```python
from build123d import *

# Parameters (mm, degrees)
F1_DEPTH = 25.4
F2_DEPTH = 31.75
F3_R     = 8.4375422203
F3_R_2   = 8.3190886378
F4_DEPTH = 74.422


with BuildPart() as f1:
    # F0 (on Front) → F1 (new body, symmetric)
    with BuildSketch(Plane.XZ):
        with BuildLine():
            Line((-29.9681008023, 26.6969427466), (-56.9970235229, 26.6969427466))
            Line((-56.9970235229, 26.6969427466), (-56.9970235229, -26.6969427466))
            Line((-56.9970235229, -26.6969427466), (56.9970235229, -26.6969427466))
            Line((56.9970235229, -26.6969427466), (56.9970235229, 26.6969427466))
            Line((56.9970235229, 26.6969427466), (29.9681008023, 26.6969427466))
            ThreePointArc((29.9681008023, 26.6969427466), (0, -3.2711580556), (-29.9681008023, 26.6969427466))
        make_face()
    extrude(amount=F1_DEPTH, both=True)

    # F0 (on Front) → F2 (join, symmetric)
    with BuildSketch(Plane.XZ):
        with BuildLine():
            Line((-19.0461007878, 26.6969427466), (-29.9681008023, 26.6969427466))
            ThreePointArc((-29.9681008023, 26.6969427466), (0, -3.2711580556), (29.9681008023, 26.6969427466))
            Line((29.9681008023, 26.6969427466), (19.0461007878, 26.6969427466))
            ThreePointArc((19.0461007878, 26.6969427466), (0, 7.6508419588), (-19.0461007878, 26.6969427466))
        make_face()
    extrude(amount=F2_DEPTH, both=True)

    # F3 (on face) → F4 (cut)
    with BuildSketch(Plane.XY.offset(26.6969427466)):
        with Locations((-38.0215607584, 0)):
            Circle(F3_R)
        with Locations((39.8610122502, 0)):
            Circle(F3_R_2)
    extrude(amount=-F4_DEPTH, mode=Mode.SUBTRACT)


solid = f1.part
```
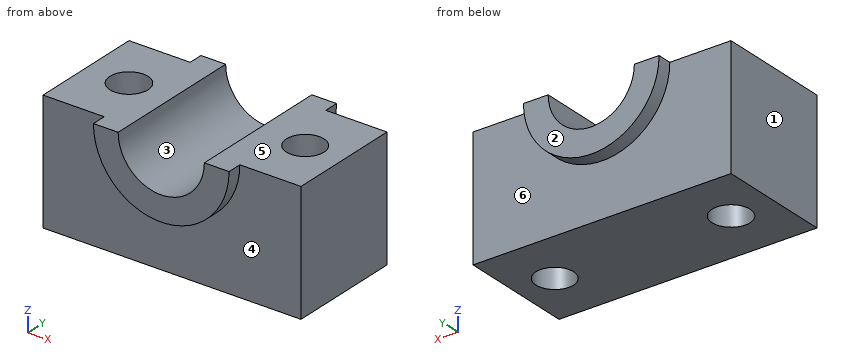
Input: part model. Units: mm. Frame: model coordinates. Face numbers are marked on the shaded views. A direction names the side the tool comes from. Round coordinates to 2 decimals unless told otherwise and drop trailing zeros. Loops run counter-clockwise (first coordinate to the right, second up) from the corner with the lowest first, then second, coordinate; pieces in that order, holes last.
1) Pull-direction query (X, two-part tool) for the marked faces 1, 2 and 3; classes: released by +X, released by -X, zero draft, split by the parting line, or undercut.
Ans:
face 1: released by -X
face 2: zero draft
face 3: undercut
2) Section query B-B on x = 0. Return the cut outline in (y, z), plus the area to 3 significant figures.
Ans:
outline: (-31.75, -3.27) - (-25.4, -3.27) - (-25.4, -26.7) - (25.4, -26.7) - (25.4, -3.27) - (31.75, -3.27) - (31.75, 7.65) - (-31.75, 7.65) - close
area: 1,880 mm2
3) Section query C-C on x = 47. Return the cut outline in (y, z).
Ans:
outline: (-25.4, -26.7) - (-4.27, -26.7) - (-4.27, 26.7) - (-25.4, 26.7) - close; (4.27, -26.7) - (25.4, -26.7) - (25.4, 26.7) - (4.27, 26.7) - close
4) Section query D-D on z = -17. Return the cut outline in (x, y).
Ans:
outline: (-57, -25.4) - (57, -25.4) - (57, 25.4) - (-57, 25.4) - close; hole circle Ø16.88 at (-38.02, 0); hole circle Ø16.64 at (39.86, 0)
5) Set-up query: the marked faces 4, 5 and 6. Return all of +Z, -Z, +X, -X, +Y, -Y with unobstructed straight access to the full face (end or side cutting, diameter ignored); none if empty.
Ans:
face 4: -Z, -Y
face 5: +Z, +X, -X, +Y, -Y
face 6: -Z, +Y
6) Section query A-A on y = 0. Return the cut outline in (x, z), plus the area to 3 significant figures.
Ans:
outline: (-57, -26.7) - (-46.46, -26.7) - (-46.46, 26.7) - (-57, 26.7) - close; (-29.58, -26.7) - (31.54, -26.7) - (31.54, 26.7) - (19.05, 26.7) arc R19.05 cw to (-19.05, 26.7) - (-29.58, 26.7) - close; (48.18, -26.7) - (57, -26.7) - (57, 26.7) - (48.18, 26.7) - close
area: 3,730 mm2
7) Pin query (flat end, axial travel): pin 1 (12 mm diameter, centred on x = -17, z = -15, fed in from +Y). Return the tip coordinate at first contact, or that it passes through.
Ans:
pin 1: stops at y = 25.4
8) Material intervals for line 1 (Y direction, x = 40.5, z = -3); line 2 (Y direction, x = 23.5, z = 0.5); line 3 (X direction, y = -1.5, z = 11.5), sorted ascending.
Ans:
line 1: y = -25.4 to -8.29, 8.29 to 25.4
line 2: y = -25.4 to 25.4
line 3: x = -57 to -46.32, -29.72 to -11.48, 11.48 to 31.68, 48.04 to 57
